```python
from build123d import *

# Parameters (mm, degrees)
SKETCH_1_W          = 40
SKETCH_1_H          = 70.5
EXTRUDE_1_DEPTH     = 9
CHAMFER_1_SIZE      = 2
FILLET_3_R          = 20
SKETCH_2_W          = 21
SKETCH_2_H          = 41
CUT_EXTRUDE_1_DEPTH = 10
SKETCH_3_W          = 2
SKETCH_3_H          = 5.5
CUT_EXTRUDE_2_DEPTH = 10
SKETCH_4_R          = 1.5
CUT_EXTRUDE_3_DEPTH = 10
SKETCH_5_R          = 1.5
CUT_EXTRUDE_4_DEPTH = 10
FILLET_4_R          = 1
CUT_EXTRUDE_5_DEPTH = 3.2
CHAMFER_2_SIZE      = 0.5


with BuildPart() as part:
    # 草图1 → 凸台-拉伸1 (new body)
    with BuildSketch(Plane.XY):
        with Locations((20, -34.75)):
            Rectangle(SKETCH_1_W, SKETCH_1_H)
    extrude(amount=EXTRUDE_1_DEPTH)

    # 倒角1
    chamfer_1_edges = [part.edges().sort_by_distance(p)[0] for p in [
        (0, 0.5, 4.5),
        (40, 0.5, 4.5),
    ]]
    chamfer(chamfer_1_edges, length=CHAMFER_1_SIZE)

    # 圆角3
    fillet_3_edges = [part.edges().sort_by_distance(p)[0] for p in [
        (0, -70, 4.5),
        (40, -70, 4.5),
    ]]
    fillet(fillet_3_edges, radius=FILLET_3_R - 0.0001)  # a hair under: the kernel refuses the full size

    # 草图2 → 切除-拉伸1 (cut)
    with BuildSketch(Plane(origin=(0, 0, 0), x_dir=(-1, 0, 0), z_dir=(0, 0, -1))):
        with Locations((-20, -40.32)):
            Rectangle(SKETCH_2_W, SKETCH_2_H)
    extrude(amount=-CUT_EXTRUDE_1_DEPTH, mode=Mode.SUBTRACT)

    # 草图3 → 切除-拉伸2 (cut)
    with BuildSketch(Plane.XY.offset(9)):
        with Locations((20, -17.07)):
            Rectangle(SKETCH_3_W, SKETCH_3_H)
        with Locations((20, -63.57)):
            Rectangle(SKETCH_3_W, SKETCH_3_H)
    extrude(amount=-CUT_EXTRUDE_2_DEPTH, mode=Mode.SUBTRACT)

    # 草图4 → 切除-拉伸3 (cut)
    with BuildSketch(Plane(origin=(0, 0, 0), x_dir=(-1, 0, 0), z_dir=(0, 0, -1))):
        with Locations((-25, -16.07)):
            Circle(SKETCH_4_R)
        with Locations((-15, -16.07)):
            Circle(SKETCH_4_R)
        with Locations((-25, -64.57)):
            Circle(SKETCH_4_R)
        with Locations((-15, -64.57)):
            Circle(SKETCH_4_R)
    extrude(amount=-CUT_EXTRUDE_3_DEPTH, mode=Mode.SUBTRACT)

    # 草图5 → 切除-拉伸4 (cut)
    with BuildSketch(Plane(origin=(0, 0, 0), x_dir=(-1, 0, 0), z_dir=(0, 0, -1))):
        with Locations((-34, -3.5)):
            Circle(SKETCH_5_R)
        with Locations((-20, -3.5)):
            Circle(SKETCH_5_R)
        with Locations((-6, -3.5)):
            Circle(SKETCH_5_R)
    extrude(amount=-CUT_EXTRUDE_4_DEPTH, mode=Mode.SUBTRACT)

    # 圆角4
    fillet_4_edges = [part.edges().sort_by_distance(p)[0] for p in [
        (21, -66.32, 4.5),
        (19, -66.32, 4.5),
        (21, -14.32, 4.5),
        (19, -14.32, 4.5),
    ]]
    fillet(fillet_4_edges, radius=FILLET_4_R - 0.0001)  # a hair under: the kernel refuses the full size

    # 草图7 → 切除-拉伸5 (cut)
    with BuildSketch(Plane(origin=(0, 0, 0), x_dir=(-1, 0, 0), z_dir=(0, 0, -1))):
        with BuildLine():
            Line((-36.9, -3.5), (-36.9, 0.5))
            Line((-36.9, 0.5), (-31.1, 0.5))
            Line((-31.1, 0.5), (-31.1, -3.5))
            ThreePointArc((-31.1, -3.5), (-34, -6.4), (-36.9, -3.5))
        make_face()
        with BuildLine():
            Line((-17.1, -3.5), (-17.1, 0.5))
            Line((-17.1, 0.5), (-22.9, 0.5))
            Line((-22.9, 0.5), (-22.9, -3.5))
            ThreePointArc((-22.9, -3.5), (-20, -6.4), (-17.1, -3.5))
        make_face()
        with BuildLine():
            Line((-3.1, -3.5), (-3.1, 0.5))
            Line((-3.1, 0.5), (-8.9, 0.5))
            Line((-8.9, 0.5), (-8.9, -3.5))
            ThreePointArc((-8.9, -3.5), (-6, -6.4), (-3.1, -3.5))
        make_face()
    extrude(amount=-CUT_EXTRUDE_5_DEPTH, mode=Mode.SUBTRACT)

    # 倒角2
    chamfer_2_edges = [part.edges().sort_by_distance(p)[0] for p in [
        (16.5, -16.07, 0),
        (26.5, -64.57, 0),
        (16.5, -64.57, 0),
        (26.5, -16.07, 0),
        (34, -6.4, 0),
        (31.1, -1.5, 0),
        (36.9, -1.5, 0),
        (20, -6.4, 0),
        (17.1, -1.5, 0),
        (22.9, -1.5, 0),
        (6, -6.4, 0),
        (3.1, -1.5, 0),
        (8.9, -1.5, 0),
    ]]
    chamfer(chamfer_2_edges, length=CHAMFER_2_SIZE)


solid = part.part
```
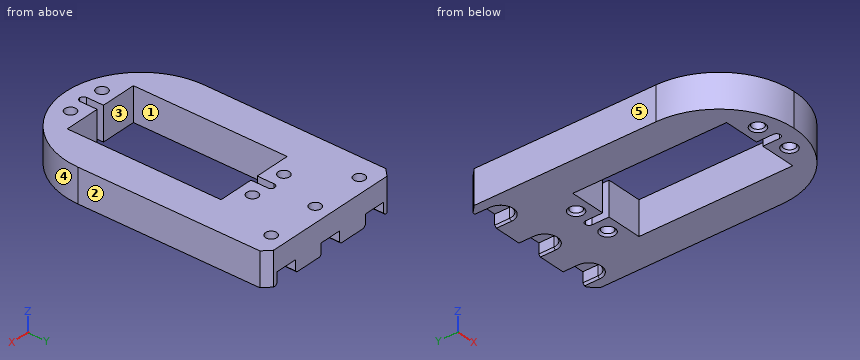
Read the model definition and answer for the solid it produces. Units are mm, in the model's axes. Face numbers are marked on the shaded views. A direction names the side the tool comes from. Coordinates: 2 decimals unless noted, no trailing zeros. Loops run counter-clockwise (first coordinate to the right, second up) from the corner with the lowest first, then second, coordinate; pieces in that order, holes last. Notation, with made-up numbers: (40, 75.5) -> (83, 75.5) arc R20 ccw to (83, 81.5) -> close; hole circle Ø11 at (42.5, -29.75). An arc over 180 degrees is marked (long way). Return JSON: item names as keys, results as strings.
Item 1: Find the intervals of material crossed by probe 1 along Y at (x, z) = (20, 6.45); probe 2 along X at (y, z) = (-49, 8); probe 3 along Y at (x, z) = (25, 4.25), in increasing order.
Answers:
{"probe 1": "y = -70 to -66.32, -14.32 to -5, -2 to 0.5", "probe 2": "x = 0 to 9.5, 30.5 to 40", "probe 3": "y = -69.36 to -66.07, -63.07 to -60.82, -19.82 to -17.57, -14.57 to 0.5"}
Item 2: For the marked faces 1 and 2, determine the directions among +Z, -Z, +X, -X, +Y, -Y from which every point of the face is accessible in a straight line to the end or side of a thin tool.
Answers:
{"face 1": "+Z, -Z", "face 2": "+Z, -Z, +X, +Y, -Y"}
Item 3: Find section D-D (z = 4.5). Count the separate pieces of the cut face and the enclosed holes in it, plus the area to 3 significant figures.
Answers:
{"separate pieces": "1", "enclosed holes": "8", "area": "1,710 mm2"}
Item 4: Flat-ended cylindrical pins translate along their axes: P1, Ø5, axis at y = -62.5, z = 3, coming from the +X side; P2, Ø3.5, axis at x = 6, y = -3.5, coming from the +Z side; P3, Ø2, axis at x = 16.5, z = 5, coming from the -Y side; P4, Ø4.5, axis at x = 6.5, y = -1.5, coming from the -Z side. Find the tip coordinate at first contact, or state that the pin passes through.
Answers:
{"P1": "stops at x = 37.32", "P2": "stops at z = 9", "P3": "stops at y = -69.84", "P4": "stops at z = 3.2"}
Item 5: Find section C-C (y = -64.57). Determine the outline of the cut face in (x, z).
Answers:
{"outline": "(6.3, 0) -> (13, 0) -> (13.5, 0.5) -> (13.5, 9) -> (6.3, 9) -> close; (16.5, 0.5) -> (17, 0) -> (19, 0) -> (19, 9) -> (16.5, 9) -> close; (21, 0) -> (23, 0) -> (23.5, 0.5) -> (23.5, 9) -> (21, 9) -> close; (26.5, 0.5) -> (27, 0) -> (33.7, 0) -> (33.7, 9) -> (26.5, 9) -> close"}
Item 6: Find section B-B (x = 11.5). Determine the outline of the cut face in (y, z).
Answers:
{"outline": "(-68.1, 0) -> (-60.82, 0) -> (-60.82, 9) -> (-68.1, 9) -> close; (-19.82, 0) -> (0.5, 0) -> (0.5, 9) -> (-19.82, 9) -> close"}
Item 7: For a pull along Y with two mould halves and no side action, classify the marked faces 3, 4 and 5 as +Y half, -Y half, draft (parallel to the pull), parting line (faces both ways), or undercut.
Answers:
{"face 3": "undercut", "face 4": "-Y half", "face 5": "draft"}
Item 8: Find section A-A (y = -36.5). Determine the outline of the cut face in (x, z).
Answers:
{"outline": "(0, 0) -> (9.5, 0) -> (9.5, 9) -> (0, 9) -> close; (30.5, 0) -> (40, 0) -> (40, 9) -> (30.5, 9) -> close"}
